from build123d import *

# Parameters (mm, degrees)
BOSS_EXTRUDE1_DEPTH  = 133.35
SKETCH2_W            = 6.06425
SKETCH2_H            = 5.11175
BOSS_EXTRUDE2_DEPTH  = 1.5875
FILLET1_R            = 3.175
FILLET1_OF_MIRROR1_R = 3.175
FILLET2_R            = 0.635
BOSS_EXTRUDE3_DEPTH  = 11.150000052


with BuildPart() as part:
    # Sketch1 → Boss-Extrude1 (new body)
    with BuildSketch(Plane.XY):
        Polygon((0.142875, 3.667125), (3.032125, 3.667125), (3.032125, 1.905), (3.032125, 0.142875), (0.142875, 0.142875), (0.142875, 1.905), align=None)
    extrude(amount=BOSS_EXTRUDE1_DEPTH)

    # Sketch2 → Boss-Extrude2 (add)
    with BuildSketch(Plane.XY.offset(133.35)):
        with Locations((1.5875, 2.69875)):
            Rectangle(SKETCH2_W, SKETCH2_H)
    boss_extrude2 = extrude(amount=BOSS_EXTRUDE2_DEPTH)

    # Fillet1
    # the kernel refuses this fillet: 3.175 mm, written as the material it takes off along each edge
    with BuildSketch(Plane(origin=(-1.444625, 5.254625, 125.4125), x_dir=(0, -1, 0), z_dir=(0, 0, 1))) as fillet1_piece_1:
        with BuildLine():
            CenterArc((FILLET1_R, FILLET1_R), FILLET1_R, 180, 90)
            Line((0, FILLET1_R), (0, 0))
            Line((0, 0), (FILLET1_R, 0))
        make_face()
    extrude(amount=17.4625, mode=Mode.SUBTRACT)
    with BuildSketch(Plane(origin=(4.619625, 5.254625, 125.4125), x_dir=(0, -1, 0), z_dir=(0, 0, 1))) as fillet1_piece_2:
        with BuildLine():
            CenterArc((FILLET1_R, -FILLET1_R), FILLET1_R, 90, 90)
            Line((0, -FILLET1_R), (0, 0))
            Line((0, 0), (FILLET1_R, 0))
        make_face()
    extrude(amount=17.4625, mode=Mode.SUBTRACT)

    # Mirror1: Boss-Extrude2 across plane
    add(boss_extrude2.mirror(Plane.XY.offset(66.675)))

    # Fillet1 of Mirror1
    # the kernel refuses this fillet: 3.175 mm, written as the material it takes off along each edge
    with BuildSketch(Plane(origin=(-1.444625, 5.254625, 7.9375), x_dir=(0, -1, 0), z_dir=(0, 0, -1))) as fillet1_of_mirror1_piece_1:
        with BuildLine():
            CenterArc((FILLET1_OF_MIRROR1_R, -FILLET1_OF_MIRROR1_R), FILLET1_OF_MIRROR1_R, 90, 90)
            Line((0, -FILLET1_OF_MIRROR1_R), (0, 0))
            Line((0, 0), (FILLET1_OF_MIRROR1_R, 0))
        make_face()
    extrude(amount=17.4625, mode=Mode.SUBTRACT)
    with BuildSketch(Plane(origin=(4.619625, 5.254625, 7.9375), x_dir=(0, -1, 0), z_dir=(0, 0, -1))) as fillet1_of_mirror1_piece_2:
        with BuildLine():
            CenterArc((FILLET1_OF_MIRROR1_R, FILLET1_OF_MIRROR1_R), FILLET1_OF_MIRROR1_R, 180, 90)
            Line((0, FILLET1_OF_MIRROR1_R), (0, 0))
            Line((0, 0), (FILLET1_OF_MIRROR1_R, 0))
        make_face()
    extrude(amount=17.4625, mode=Mode.SUBTRACT)

    # Fillet2
    fillet2_edges = [part.edges().sort_by_distance(p)[0] for p in [
        (3.032125, 3.667125, 66.675),
        (0.142875, 3.667125, 66.675),
    ]]
    fillet(fillet2_edges, radius=FILLET2_R)

    # Sketch3 → Boss-Extrude3 (add)
    with BuildSketch(Plane.XZ.offset(-0.142875)):
        Polygon((-1.444625, 134.9375), (4.619625, 134.9375), (4.619625, 133.35), (3.032125, 133.35), (3.032125, 0), (4.619625, 0), (4.619625, -1.5875), (-1.444625, -1.5875), (-1.444625, 0), (0.142875, 0), (0.142875, 133.35), (-1.444625, 133.35), align=None)
    extrude(amount=BOSS_EXTRUDE3_DEPTH)


solid = part.part
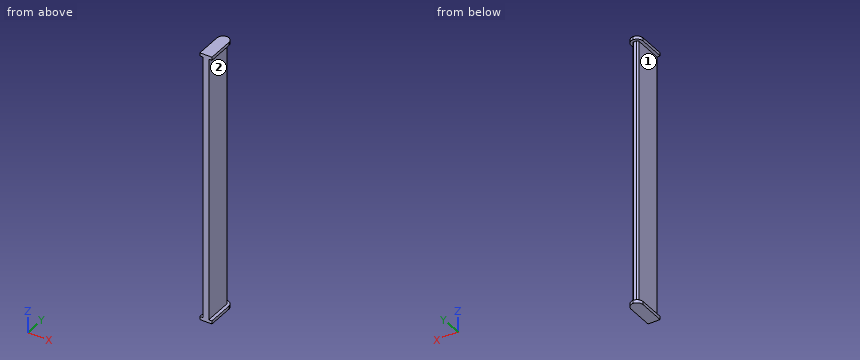
Geometry: final body of the model. Coordinates: model frame, mm. Face numbers are marked on the shaded views. A direction names the side the tool comes from. Round coordinates to 2 decimals unless told otherwise and drop trailing zeros. Write each loop counter-clockwise with the first axis right and the second up, starting at its lowest first coordinate (ties: lowest second). Pieces come first, ordered by that corner, then holes. Notation, with made-up numbers: M 87.5,-37.5 L 135.5,-37.5 A11 ccw 135.5,-25.5 Z; hole C 33.5,48.25 d10. An arc over 180 degrees is marked long. Write item = value, one per line.
Item 1: Section query B-B on z = 120.5. Return loops of the section in (x, y) (3 decimals).
Findings:
outline = M 0.143,-11.007 L 3.032,-11.007 L 3.032,3.032 A0.635 ccw 2.397,3.667 L 0.778,3.667 A0.635 ccw 0.143,3.032 Z
Item 2: Access query for the marked faces 1 and 2. Directions: +Z, -Z, +X, -X, +Y, -Y. A direction counts if a zero-diameter tool reaches every point of the face in a straight line with its end or side. Return the directions, or none.
Findings:
face_1 = -X, +Y, -Y
face_2 = +X, +Y, -Y
Item 3: Material intervals for line 1 along Z through (x, y) = (-0.75, -3.75); line 2 along X through (y, z) = (-2.25, 57); line 3 along Y through (x, z) = (2.5, 33), sorted ascending. Write a range as [from, to].
Findings:
line_1 = [-1.59, 0], [133.35, 134.94]
line_2 = [0.14, 3.03]
line_3 = [-11.01, 3.66]
Item 4: Pin query (flat end, axial travel): P1, Ø7, axis at y = -0.5, z = 49, coming from the +X side; P2, Ø0.5, axis at x = 1.5, z = 58, coming from the +Y side; P3, Ø4, axis at y = -2, z = 94, coming from the -X side. Return the tip coordinate at first contact, or that it passes through.
Findings:
P1 = 3.03
P2 = 3.67
P3 = 0.14
Item 5: Section query A-A on y = -4.25. Return loops of the section in (x, z).
Findings:
outline = M -1.44,-1.59 L 4.62,-1.59 L 4.62,0 L 3.03,0 L 3.03,133.35 L 4.62,133.35 L 4.62,134.94 L -1.44,134.94 L -1.44,133.35 L 0.14,133.35 L 0.14,0 L -1.44,0 Z
